```python
from build123d import *

# Parameters (mm, degrees)
F0_W     = 167.511746
F0_H     = 106.832422
F1_DEPTH = 103.378
F2_R     = 19.899067
F3_DEPTH = 229.362
F4_W     = 88.121988
F4_H     = 47.376074
F5_DEPTH = 133.096


with BuildPart() as f1:
    # F0 (on Right) → F1 (new body)
    with BuildSketch(Plane.YZ):
        Rectangle(F0_W, F0_H)
    extrude(amount=F1_DEPTH)

    # F2 (on face) → F3 (cut)
    with BuildSketch(Plane.XZ.offset(83.755873)):
        with Locations((44.885427, 0)):
            Circle(F2_R)
    extrude(amount=-F3_DEPTH, mode=Mode.SUBTRACT)

    # F4 (on face) → F5 (cut)
    with BuildSketch(Plane.YZ.offset(103.378)):
        with Locations((0, 53.416211)):
            Rectangle(F4_W, F4_H)
    extrude(amount=-F5_DEPTH, mode=Mode.SUBTRACT)


solid = f1.part
```
Here's how the part is built. I have some questions about the finished solid (model axes, mm). A direction names the side the tool comes from. Round coordinates to 2 decimals unless told otherwise and drop trailing zeros. Write each loop counter-clockwise with the first axis right and the second up, starting at its lowest first coordinate (ties: lowest second). Pieces come first, ordered by that corner, then holes.
Q1. Which directions (+Z, -Z, +X, -X, +Y, -Y) give clear straight access to the entire face, cutting with the end or side of a thin tool? Please do faces 1 (the flat face through (52, -1, 29.728)), 2 (the flat face through (51, 64, 53.416)).
Q2. If we mould it in two halves opening along Y, with no side actions, what happens to faces 3 (the flat face through (62, 83.756, 11)), 4 (the flat face through (52, 44.061, 41)), 5 (the cylindrical face through (63.866, -1.173, 5.977))? For each: +Y half, -Y half, draft (parallel to the pull), parting line (faces both ways), or undercut.
Q3. Please list where these lines run through material, in increasing order: probe 1 along Y at (x, z) = (46, 40.5); probe 2 along Z at (x, y) = (44.5, 6); probe 3 along X at (y, z) = (-26.5, 9).
Q4. If we section it at B-B on x = 49.5: Write out the boundary of the cut face in (y, z).
Q5. If we section it at D-D on x = 19.5: Write out the boundary of the cut face in (y, z).
Q6. If we section it at A-A on z = 38: Write out the boundary of the cut face in (x, y).
Q7. If we section it at C-C on y = -23: Write out the boundary of the cut face in (x, z), plus the area to 3 significant figures.
Answer below:
1. face 1: +Z, +X, -X
1. face 2: +Z, +X, -X, +Y, -Y
2. face 3: +Y half
2. face 4: undercut
2. face 5: draft
3. probe 1: y = -83.76 to -44.06, 44.06 to 83.76
3. probe 2: z = -53.42 to -19.9, 19.9 to 29.73
3. probe 3: x = 0 to 27.14, 62.63 to 103.38
4. outline: (-83.76, -53.42) - (83.76, -53.42) - (83.76, -19.36) - (-83.76, -19.36) - close; (-83.76, 19.36) - (83.76, 19.36) - (83.76, 53.42) - (44.06, 53.42) - (44.06, 29.73) - (-44.06, 29.73) - (-44.06, 53.42) - (-83.76, 53.42) - close
5. outline: (-83.76, -53.42) - (83.76, -53.42) - (83.76, 53.42) - (44.06, 53.42) - (44.06, 29.73) - (-44.06, 29.73) - (-44.06, 53.42) - (-83.76, 53.42) - close
6. outline: (0, -83.76) - (103.38, -83.76) - (103.38, -44.06) - (0, -44.06) - close; (0, 44.06) - (103.38, 44.06) - (103.38, 83.76) - (0, 83.76) - close
7. outline: (0, -53.42) - (103.38, -53.42) - (103.38, 29.73) - (0, 29.73) - close; hole circle Ø39.8 at (44.89, 0)
7. area: 7,350 mm2
